Input: dimensioned drawing with shaded views. Units: mm. Origin: part minimum x, y, z. A direction names the side the tool comes from. Round coordinates to 2 decimals unless told otherwise and drop trailing zeros. Loops run counter-clockwise (first coordinate to the right, second up) from the corner with the lowest first, then second, coordinate; pieces in that order, holes last. Notation, with made-up numbers: (-30.75, 74) -> (7.25, 74) arc R13 ccw to (7.25, 89) -> close; hole circle Ø1 at (0, 34.25). An arc over 180 degrees is marked (long way). Answer as a JSON object with one key per item and string values.
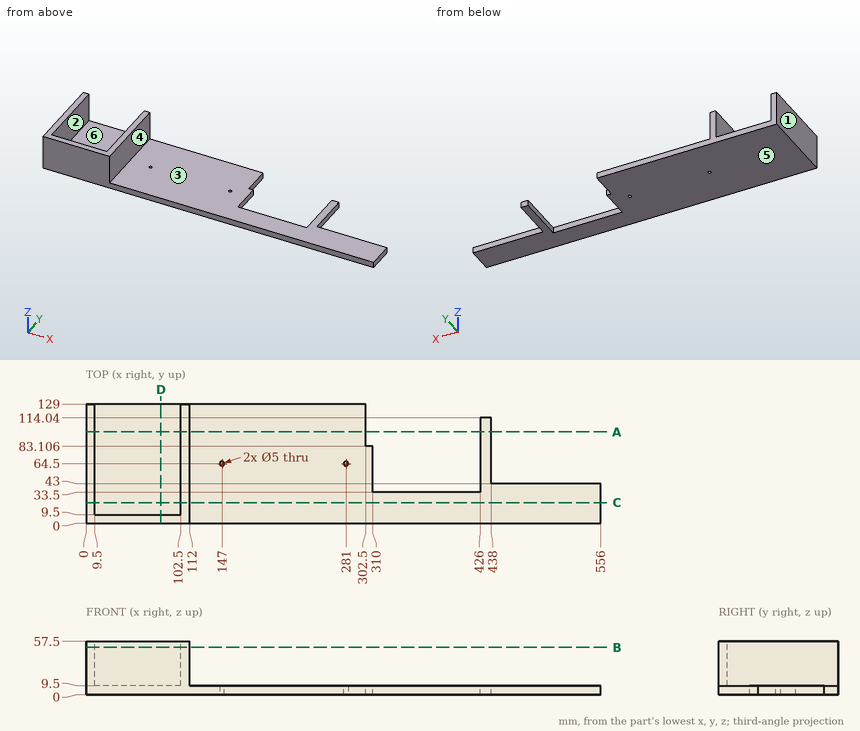
1) Section A-A, the plane y = 99. Output: boundary loops of the cut face in (x, z), plus the area to 3 significant figures.
Output:
{"outline": "(0, 0) -> (302.5, 0) -> (302.5, 9.5) -> (112, 9.5) -> (112, 57.5) -> (102.5, 57.5) -> (102.5, 9.5) -> (9.5, 9.5) -> (9.5, 57.5) -> (0, 57.5) -> close; (426, 0) -> (438, 0) -> (438, 9.5) -> (426, 9.5) -> close", "area": "3,900 mm^2"}
2) Section C-C, the plane y = 22.5. Output: boundary loops of the cut face in (x, z).
Output:
{"outline": "(0, 0) -> (556, 0) -> (556, 9.5) -> (112, 9.5) -> (112, 57.5) -> (102.5, 57.5) -> (102.5, 9.5) -> (9.5, 9.5) -> (9.5, 57.5) -> (0, 57.5) -> close"}
3) Section B-B, the plane z = 51. Output: boundary loops of the cut face in (x, y).
Output:
{"outline": "(0, 0) -> (112, 0) -> (112, 129) -> (102.5, 129) -> (102.5, 9.5) -> (9.5, 9.5) -> (9.5, 129) -> (0, 129) -> close"}
4) Ray query, probe 1 along X at (y, z) = (52, 38.5); probe 2 along Y at (x, z) = (147, 2); probe 3 along X at (y, z) = (89.5, 8). Return the intervals inside material, ascending.
Output:
{"probe 1": "x = 0 to 9.5, 102.5 to 112", "probe 2": "y = 0 to 62, 67 to 129", "probe 3": "x = 0 to 302.5, 426 to 438"}
5) Contact query for flat-ended pins moving along their axis: P1, Ø5, axis at y = 94.5, z = 2.5, coming from the +X side; P2, Ø3, axis at y = 57.5, z = 13, coming from the +X side; P3, Ø7.5, axis at x = 430.5, z = 7, coming from the +Y side; P4, Ø4, axis at x = 147, y = 64.5, coming from the -Z side. Output: stop coordinate, or through.
Output:
{"P1": "stops at x = 438", "P2": "stops at x = 112", "P3": "stops at y = 114.04", "P4": "passes through"}
6) Section D-D, the plane x = 81. Output: boundary loops of the cut face in (y, z).
Output:
{"outline": "(0, 0) -> (129, 0) -> (129, 9.5) -> (9.5, 9.5) -> (9.5, 57.5) -> (0, 57.5) -> close"}
7) Reachability of the marked faces 5 and 6 from +Z, -Z, +X, -X, +Y, -Y: full face, straight path, thin tool, end or side. Return the list, or none.
Output:
{"face 5": "-Z, +X, -X, +Y, -Y", "face 6": "+Z, +Y"}
8) Draft query along X for the marked faces 1, 2, 3 and 4. Return one class per face: +X half, -X half, draft (parallel to the pull), parting line (faces both ways), or undercut.
Output:
{"face 1": "-X half", "face 2": "undercut", "face 3": "draft", "face 4": "+X half"}
